```python
from build123d import *

# Parameters (mm, degrees)
SKETCH1_W           = 50
SKETCH1_H           = 42.5
BOSS_EXTRUDE1_DEPTH = 8
CUT_EXTRUDE1_DEPTH  = 6
SKETCH3_R           = 2.25
CUT_EXTRUDE2_DEPTH  = 34.772214911


with BuildPart() as part:
    # Sketch1 → Boss-Extrude1 (new body)
    with BuildSketch(Plane.XY):
        Rectangle(SKETCH1_W, SKETCH1_H)
    extrude(amount=BOSS_EXTRUDE1_DEPTH)

    # Sketch2 → Cut-Extrude1 (cut)
    with BuildSketch(Plane.XY.offset(8)):
        with BuildLine():
            Line((-3.292893219, -3.8), (3.292893219, -3.8))
            Line((3.292893219, -3.8), (3.792817713, -4.299924494))
            Line((3.792817713, -4.299924494), (9.707031275, -4.299924494))
            Line((9.707031275, -4.299924494), (10.499848989, -3.507106781))
            Line((10.499848989, -3.507106781), (10.499848989, -0.890716475))
            Line((10.499848989, -0.890716475), (5.426401458, 2.661749731))
            ThreePointArc((5.426401458, 2.661749731), (5.112967061, 3.019153162), (4.999977894, 3.480901775))
            Line((4.999977894, 3.480901775), (4.999977894, 5.699901775))
            ThreePointArc((4.999977894, 5.699901775), (5.292871113, 6.407008557), (5.999977894, 6.699901775))
            Line((5.999977894, 6.699901775), (15.207084675, 6.699901775))
            Line((15.207084675, 6.699901775), (15.999902388, 7.492719488))
            Line((15.999902388, 7.492719488), (15.999902388, 14.906933051))
            Line((15.999902388, 14.906933051), (15.207084675, 15.699750764))
            Line((15.207084675, 15.699750764), (7.165888575, 15.699750764))
            Line((7.165888575, 15.699750764), (6.544410681, 14.199370403))
            Line((6.544410681, 14.199370403), (-6.544410681, 14.199370403))
            Line((-6.544410681, 14.199370403), (-7.165888575, 15.699750764))
            Line((-7.165888575, 15.699750764), (-15.207084675, 15.699750764))
            Line((-15.207084675, 15.699750764), (-15.999902388, 14.906933051))
            Line((-15.999902388, 14.906933051), (-15.999902388, 7.492719488))
            Line((-15.999902388, 7.492719488), (-15.207084675, 6.699901775))
            Line((-15.207084675, 6.699901775), (-5.999977894, 6.699901775))
            ThreePointArc((-5.999977894, 6.699901775), (-5.292871113, 6.407008557), (-4.999977894, 5.699901775))
            Line((-4.999977894, 5.699901775), (-4.999977894, 3.480901775))
            ThreePointArc((-4.999977894, 3.480901775), (-5.112967061, 3.019153162), (-5.426401458, 2.661749731))
            Line((-5.426401458, 2.661749731), (-10.499848989, -0.890716475))
            Line((-10.499848989, -0.890716475), (-10.499848989, -3.507106781))
            Line((-10.499848989, -3.507106781), (-9.707031275, -4.299924494))
            Line((-9.707031275, -4.299924494), (-3.792817713, -4.299924494))
            Line((-3.792817713, -4.299924494), (-3.292893219, -3.8))
        make_face()
    extrude(amount=-CUT_EXTRUDE1_DEPTH, mode=Mode.SUBTRACT)

    # Sketch3 → Cut-Extrude2 (cut, through all)
    with BuildSketch(Plane.XY.offset(8)):
        with Locations((-15, -11.25)):
            Circle(SKETCH3_R)
        with Locations((15, -11.25)):
            Circle(SKETCH3_R)
    extrude(amount=-CUT_EXTRUDE2_DEPTH, mode=Mode.SUBTRACT)


solid = part.part
```
Can you work these out from the model? Positions are in its coordinate system, mm. A direction names the side the tool comes from. Give positions to 0.01 mm unless a question says otherwise; leave off trailing zeros. Loops run counter-clockwise (first coordinate to the right, second up) from the corner with the lowest first, then second, coordinate; pieces in that order, holes last. Notation, with made-up numbers: M 45.25,9.25 L 89.25,9.25 A15 ccw 89.25,34.25 Z; hole C 15.5,-3 d6. An arc over 180 degrees is marked long. Use CSV: the item, a comma, the result in double quotes. Start each with the question number.
1. Imagine slicing it at A-A, the plane y = -11.25. Write out the boundary of the cut face in (x, z), plus the area to 3 significant figures.
2. Imagine slicing it at B-B, the plane x = 12. Write out the boundary of the cut face in (y, z), plus the area to 3 significant figures.
3. For P1, Ø6, axis at x = 15, y = -11.25, coming from the +Z side; P2, Ø2.5, axis at x = -15, y = -11.25, coming from the +Z side, each with a flat end and sliding along its axis, tell me the tip position at first contact or that it passes through.
4. On a 3-axis mill with a long thin cutter (end or side, diameter ignored), from which of +Z, -Z, +X, -X, +Y, -Y can I reach the whole of each face in a straight line? I mean faces 4 (the face through (-16, 11, 5)), 5 (the face through (16.21, -9.353, 4.056)). Say none if no direction works.
5. If we mould it in two halves opening along Y, with no side actions, what happens to faces 1 (the face through (10.5, -2, 5)), 2 (the face through (25, 0, 4)), 3 (the face through (0, -21.25, 4))? For each: released by +Y, released by -Y, zero draft, split by the parting line, or undercut.
6. If I drill on L1, parallel to Y at x = 15, z = 6.25; L2, parallel to Y at x = -4.5, z = 4.75; L3, parallel to X at y = 9.5, z = 7.75, over which ranges is the centre line in solid material (lowest first)?
7. Imagine slicing it at C-C, the plane z = 6.25. Count the separate pieces of the cut face and the enclosed holes in it, plus the area to 3 significant figures.
8. Imagine slicing it at D-D, the plane y = 4.5. Write out the boundary of the cut face in (x, z).
Response values:
1,outline,"M -25,0 L -17.25,0 L -17.25,8 L -25,8 Z; M -12.75,0 L 12.75,0 L 12.75,8 L -12.75,8 Z; M 17.25,0 L 25,0 L 25,8 L 17.25,8 Z"
1,area,"328 mm^2"
2,outline,"M -21.25,0 L 21.25,0 L 21.25,8 L 15.7,8 L 15.7,2 L 6.7,2 L 6.7,8 L -21.25,8 Z"
2,area,"286 mm^2"
3,P1,"z = 8"
3,P2,"through"
4,face 4,"+Z"
4,face 5,"+Z, -Z"
5,face 1,"undercut"
5,face 2,"zero draft"
5,face 3,"released by -Y"
6,L1,"-21.25 to -13.5, -9 to 6.7, 15.7 to 21.25"
6,L2,"-21.25 to -4.3, 14.2 to 21.25"
6,L3,"-25 to -16, 16 to 25"
7,separate pieces,"1"
7,enclosed holes,"3"
7,area,"1,660 mm^2"
8,outline,"M -25,0 L 25,0 L 25,8 L 5,8 L 5,2 L -5,2 L -5,8 L -25,8 Z"
